Part model, mm, in its own coordinate system. A direction names the side the tool comes from. Round coordinates to 2 decimals unless told otherwise and drop trailing zeros. Loops run counter-clockwise (first coordinate to the right, second up) from the corner with the lowest first, then second, coordinate; pieces in that order, holes last. Notation, with made-up numbers: (26, 78) -> (64, 78) arc R16 cw to (64, 105) -> close; hole circle Ø6 at (76, 16). An arc over 180 degrees is marked (long way). Use a Markdown table: item, result. Add a question column.
Item 1: Cut at A-A, the plane x = -9. List the corners of the cut face in (y, z), plus the area to 3 significant figures.
Item 2: Flat gauge pin, fed straight in: pin 1 (1.5 mm diameter, centred on x = -3, z = -1, fed in from -Y). Where does the tip first touch, or does it go through?
Item 3: Which spindle directions (+Z, -Z, +X, -X, +Y, -Y) get a long thin tool onto all of the face, cutting with end or side? Do faces 1 (the face through (-26, 1, 0)), 2 (the face through (0, 2, 0)), 3 (the face through (25, 1, 0)). Say none if no direction does.
Item 4: Probe line 1 (Z direction, x = 3, y = 0.1); line 2 (Y direction, x = -15, z = -0.5); line 3 (Z direction, x = -5, y = 0.45). List the from-to ranges inside material, lowest first. Write a range as [from, to].
```python
from build123d import *

# Parameters (mm, degrees)
CHAMFER1_SIZE = 0.075


with BuildPart() as part:
    # Sketch1 → Revolve1 (revolve)
    with BuildSketch(Plane(origin=(0, 0, 0), x_dir=(1, 0, 0), z_dir=(0, 1, 0)), mode=Mode.PRIVATE) as revolve1_sk:
        with BuildLine():
            Line((-30, 0), (30, 0))
            Line((30, 0), (30, 1))
            Line((30, 1), (21, 1))
            ThreePointArc((21, 1), (19.178802434, 1.167873273), (17.418979879, 1.665835704))
            ThreePointArc((17.418979879, 1.665835704), (16.535774215, 1.915749105), (15.621766151, 2))
            Line((15.621766151, 2), (-15.621766151, 2))
            ThreePointArc((-15.621766151, 2), (-16.535774215, 1.915749105), (-17.418979879, 1.665835704))
            ThreePointArc((-17.418979879, 1.665835704), (-19.178802434, 1.167873273), (-21, 1))
            Line((-21, 1), (-30, 1))
            Line((-30, 1), (-30, 0))
        make_face()
    revolve(revolve1_sk.sketch.rotate(Axis((-30, 0, 0), (1, 0, 0)), 180), axis=Axis((-30, 0, 0), (1, 0, 0)))

    # Chamfer1
    chamfer1_edges = [part.edges().sort_by_distance(p)[0] for p in [
        (30, 0, -1),
        (-30, 0, -1),
    ]]
    chamfer(chamfer1_edges, length=CHAMFER1_SIZE)


solid = part.part
```
A:
| question | item | result |
|---|---|---|
| 1 | outline | circle Ø4 at (0, 0) |
| 1 | area | 12.6 mm^2 |
| 2 | pin 1 | stops at y = -1.98 |
| 3 | face 1 | -X |
| 3 | face 2 | +X, -X |
| 3 | face 3 | +X |
| 4 | line 1 | z = [-2, 2] |
| 4 | line 2 | y = [-1.94, 1.94] |
| 4 | line 3 | z = [-1.95, 1.95] |
